Autodesk Inventor part; units mm, degrees
ref_plane "YZ Plane" through (0, 0, 0) normal (1, 0, 0) x (0, 1, 0)
ref_plane "XZ Plane" through (0, 0, 0) normal (0, 1, 0) x (-1, 0, 0)
ref_plane "XY Plane" through (0, 0, 0) normal (0, 0, 1) x (1, 0, 0)
sketch "Эскиз1" plane through (0, 0, 0) normal (0, 1, 0) x (-1, 0, 0)
  line L0 (-14, 14) -> (14, 14)
  line L1 (14, 14) -> (14, -14)
  line L2 (14, -14) -> (-14, -14)
  line L3 (-14, -14) -> (-14, 14)
  line L4 (-14, 14) -> (14, -14) construction
  line L5 (14, 14) -> (-14, -14) construction
  point P0 (0, 0)
  dimension "d0" = 28
  dimension "d1" = 28
extrude "Выдавливание1" add sketch "Эскиз1" along normal blind 56
sketch "Эскиз2" plane through (0, 0, 0) normal (0, -1, 0) x (1, 0, 0)
  circle A0 centre (0, 0) radius 4
extrude "Выдавливание2" cut sketch "Эскиз2" against normal blind 32
sketch "Эскиз3" plane through (-14, 0, -14) normal (-1, 0, 0) x (0, 0, 1)
  circle A0 centre (14, 46) radius 4
  point P0 (14, 0)
extrude "Выдавливание3" cut sketch "Эскиз3" against normal through all
sketch "Эскиз4" plane through (14, 0, 14) normal (1, 0, 0) x (0, 0, -1)
  circle A0 centre (14, 46) radius 4
  line L0 (6.2058, 46) -> (10.1029, 52.75)
  line L1 (10.1029, 52.75) -> (17.8971, 52.75)
  line L2 (17.8971, 52.75) -> (21.7942, 46)
  line L3 (21.7942, 46) -> (17.8971, 39.25)
  line L4 (17.8971, 39.25) -> (10.1029, 39.25)
  line L5 (10.1029, 39.25) -> (6.2058, 46)
  line L6 (0, 56) -> (28, 56)
  point P0 (14, 0)
  dimension "d8" = 13.5
extrude "Выдавливание4" cut sketch "Эскиз4" against normal blind 10
chamfer "Фаска1" distance 2 angle 45 6 edges at (14, 39.25, 0) (14, 42.625, -5.8457) (14, 49.375, -5.8457) (14, 52.75, 0) (14, 49.375, 5.8457) (14, 42.625, 5.8457)
ref_plane "РабПлоскость1" through (0, 22, 0) normal (0, -1, 0) x (1, 0, 0)
sketch "Эскиз5" plane through (0, 22, 0) normal (0, -1, 0) x (1, 0, 0)
  line L0 (0, 8.0829) -> (7, 4.0415)
  line L1 (7, 4.0415) -> (7, -4.0415)
  line L2 (7, -4.0415) -> (0, -8.0829)
  line L3 (0, -8.0829) -> (-7, -4.0415)
  line L4 (-7, -4.0415) -> (-7, 4.0415)
  line L5 (-7, 4.0415) -> (0, 8.0829)
  line L6 (0, 8.0829) -> (-14, 8.0829)
  line L7 (-14, -14) -> (-14, 14)
  line L8 (0, -8.0829) -> (-14, -8.0829)
  line L9 (-14, 8.0829) -> (-14, -8.0829)
  point P0 (0, 0)
  point P1 (0, 0)
  dimension "d15" = 14
extrude "Выдавливание5" cut sketch "Эскиз5" along normal mid plane 10
chamfer "Фаска2" distance 2 angle 45 4 edges at (-14, 27, 0) (-14, 22, 8.0829) (-14, 17, 0) (-14, 22, -8.0829)
sketch "Эскиз6" plane through (-14, 0, -14) normal (-1, 0, 0) x (0, 0, 1)
  line L0 (28, 0) -> (28, 56)
  line L1 (0, 0) -> (0, 56)
  line L2 (28, 0) -> (0, 0)
  line L3 (0, 0) -> (0, 30)
  line L4 (0, 30) -> (28, 30)
  line L5 (28, 30) -> (28, 0)
  line L6 (24.0829, 15) -> (24.0829, 29)
  line L7 (3.9171, 15) -> (24.0829, 15)
  line L8 (3.9171, 29) -> (3.9171, 15)
  line L9 (24.0829, 29) -> (3.9171, 29)
  point P0 (14, 0)
  point P1 (28, 30)
  dimension "d21" = 30
extrude "Выдавливание6" add sketch "Эскиз6" along normal blind 2
sketch "Эскиз7" plane through (-14, 56, 14) normal (0, 0, 1) x (1, 0, 0)
  circle A0 centre (14, -18) radius 1.85
  point P0 (14, -56)
extrude "Выдавливание7" cut sketch "Эскиз7" against normal blind 12
mirror "Зеркальное отражение1" about plane through (0, 0, 0) normal (0, 0, 1) of "Выдавливание7"
sketch "Эскиз8" plane through (-14, 56, 14) normal (0, 0, 1) x (1, 0, 0)
  circle A0 centre (14, -18) radius 1.85
  line L0 (9.6699, -18) -> (11.8349, -14.25)
  line L1 (11.8349, -14.25) -> (16.1651, -14.25)
  line L2 (16.1651, -14.25) -> (18.3301, -18)
  line L3 (18.3301, -18) -> (16.1651, -21.75)
  line L4 (16.1651, -21.75) -> (11.8349, -21.75)
  line L5 (11.8349, -21.75) -> (9.6699, -18)
  point P0 (14, -56)
  dimension "d26" = 7.5
extrude "Выдавливание8" cut sketch "Эскиз8" against normal blind 4 contours A0 | L0 L1 L2 L3 L4 L5
mirror "Зеркальное отражение2" about plane through (0, 0, 0) normal (0, 0, 1) of "Выдавливание8"
equation "\"d1\" = d0"
equation "\"d2\" = 2 * d0"
properties part number "000.001.001 - Уголок" material "Пластик АБС"
Verification items for the finished model (mm, model axes). A direction names the side the tool comes from. Coordinates: 2 decimals unless noted, no trailing zeros. Order: outer loops, then holes, each group sorted by start corner. A loop starts at its lowest first (then second) coordinate and runs counter-clockwise, first axis right, second up. Notation, with made-up numbers: M 88.25,58.25 L 129.25,58.25 A18 cw 129.25,86.25 Z; hole C -37,8 d4. An arc over 180 degrees is marked long. Return JSON: item names as keys, results as strings.
1) Cross-section at C-C, the plane y = 45. Record the boundary of the cut face in (x, z).
Answer list:
{"outline": "M -14,-14 L 14,-14 L 14,-9.53 L 12,-7.22 L 4,-7.22 L 4,-3.87 L -14,-3.87 Z; M -14,3.87 L 4,3.87 L 4,7.22 L 12,7.22 L 14,9.53 L 14,14 L -14,14 Z"}
2) Release check for a two-part mould opening along Z. For faces 4 (the flat face through (-12.986, 21.902, -9.069)), 5 (the flat face through (-3.26, 39.85, 12.03)), 6 (the flat face through (0, 38, -2)) record: +Z half, -Z half, draft (parallel to the pull), parting line (faces both ways), or undercut.
Answer list:
{"face 4": "undercut", "face 5": "draft", "face 6": "-Z half"}
3) Cross-section at D-D, the plane z = -11.75. Record the boundary of the cut face in (x, y).
Answer list:
{"outline": "M -16,0 L 14,0 L 14,56 L -14,56 L -14,30 L -16,30 Z; hole M -4.33,38 L -2.17,34.25 L 2.17,34.25 L 4.33,38 L 2.17,41.75 L -2.17,41.75 Z"}
4) Thickness scan on L1, parallel to Y at x = 0, z = 6.5; L2, parallel to Y at x = -5.5, z = 0; L3, parallel to Z at x = -6, y = 20. Record the ranges inside material, lowest first. Write a range as [from, to].
Answer list:
{"L1": "[0, 17], [27, 36.15], [39.85, 56]", "L2": "[0, 17], [27, 42], [50, 56]", "L3": "[-14, -8.08], [8.08, 14]"}
5) Cross-section at A-A, the plane z = 0. Count the separate pieces of the cut face and the enclosed holes in it, and give its area (3 significant figures).
Answer list:
{"separate pieces": "3", "enclosed holes": "0", "area": "927 mm2"}
6) Cross-section at B-B, the plane x = 10. Record the boundary of the cut face in (y, z), and give its area (3 significant figures).
Answer list:
{"outline": "M 0,-14 L 56,-14 L 56,14 L 0,14 Z; hole M 39.25,-3.9 L 46,-7.79 L 52.75,-3.9 L 52.75,3.9 L 46,7.79 L 39.25,3.9 Z", "area": "1,410 mm2"}
7) Access from +Z, -Z, +X, -X, +Y, -Y to the whole of each face (thin tool, end or side, straight path). Record for faces 1 (the flat face through (3.26, 36.15, 12.03)), 2 (the flat face through (-3.26, 36.15, -12.03)), 3 (the flat face through (3.45, 22.07, 6.09)).
Answer list:
{"face 1": "+Z", "face 2": "-Z", "face 3": "-X"}
8) Gauge pin test, flat ends, axial feed: pin 1 (2 mm diameter, centred on x = 0, y = 38, fed in from +Z); pin 2 (9 mm diameter, centred on y = 46, z = 0, fed in from +X); pin 3 (6 mm diameter, centred on x = 0, y = 38, fed in from -Z). Record the tip position at first contact, or that the pin passes through.
Answer list:
{"pin 1": "z = 2", "pin 2": "x = 4", "pin 3": "z = -10"}
